from build123d import *

# Parameters (mm, degrees)
SKETCH_3_R          = 13
EXTRUDE_1_DEPTH     = 5
CUT_EXTRUDE_2_DEPTH = 2.5
SKETCH_4_R          = 10
EXTRUDE_2_DEPTH     = 15


with BuildPart() as part:
    # ｽｹｯﾁ3 → ﾎﾞｽ - 押し出し1 (new body)
    with BuildSketch(Plane.XY):
        Circle(SKETCH_3_R)
    extrude(amount=EXTRUDE_1_DEPTH)

    # ｽｹｯﾁ2 → ｶｯﾄ - 押し出し2 (cut)
    with BuildSketch(Plane.XY):
        with BuildLine():
            Line((3.75, 6.495190528), (2.463350586, 13.926501921))
            ThreePointArc((2.463350586, 13.926501921), (0, 16), (-2.463350586, 13.926501921))
            Line((-2.463350586, 13.926501921), (-3.75, 6.495190528))
            Line((-3.75, 6.495190528), (-10.829029157, 9.096575147))
            ThreePointArc((-10.829029157, 9.096575147), (-13.856406461, 8), (-13.292379743, 4.829926775))
            Line((-13.292379743, 4.829926775), (-7.5, 0))
            Line((-7.5, 0), (-13.292379743, -4.829926775))
            ThreePointArc((-13.292379743, -4.829926775), (-13.856406461, -8), (-10.829029157, -9.096575147))
            Line((-10.829029157, -9.096575147), (-3.75, -6.495190528))
            Line((-3.75, -6.495190528), (-2.463350586, -13.926501921))
            ThreePointArc((-2.463350586, -13.926501921), (0, -16), (2.463350586, -13.926501921))
            Line((2.463350586, -13.926501921), (3.75, -6.495190528))
            Line((3.75, -6.495190528), (10.829029157, -9.096575147))
            ThreePointArc((10.829029157, -9.096575147), (13.856406461, -8), (13.292379743, -4.829926775))
            Line((13.292379743, -4.829926775), (7.5, 0))
            Line((7.5, 0), (13.292379743, 4.829926775))
            ThreePointArc((13.292379743, 4.829926775), (13.856406461, 8), (10.829029157, 9.096575147))
            Line((10.829029157, 9.096575147), (3.75, 6.495190528))
        make_face()
    extrude(amount=CUT_EXTRUDE_2_DEPTH, mode=Mode.SUBTRACT)

    # ｽｹｯﾁ4 → ﾎﾞｽ - 押し出し2 (add)
    with BuildSketch(Plane.XY.offset(5)):
        Circle(SKETCH_4_R)
    extrude(amount=EXTRUDE_2_DEPTH)

    # ｽｹｯﾁ5 → 回転1 (revolve)
    with BuildSketch(Plane(origin=(0, 0, 0), x_dir=(1, 0, 0), z_dir=(0, 1, 0))):
        Polygon((0, -20), (25, -20), (25, -22), (10, -22), (10, -30), (25, -30), (25, -32), (0, -32), align=None)
    revolve(axis=Axis((0, 0, 0), (0, 0, 1)))


solid = part.part
Check sheet for the modelled part. Datum: model origin and axes. Units: mm. A direction names the side the tool comes from. Round coordinates to 2 decimals unless told otherwise and drop trailing zeros. Loops run counter-clockwise (first coordinate to the right, second up) from the corner with the lowest first, then second, coordinate; pieces in that order, holes last. Notation, with made-up numbers: M 6.5,49.5 L 24.5,49.5 A21 ccw 24.5,53.5 Z; hole C 65,72.25 d8. An arc over 180 degrees is marked long. One line per question, with ' | ' between items. Start each with the question number.
Item 1: Set-up check for faces 4 (the face through (0, -11, 30)), 5 (the face through (6.67, -7.57, 1.23)), 6 (the face through (3.218, 9.565, 1.232)): record each of +Z, -Z, +X, -X, +Y, -Y from which the full face is reachable in a straight line by a thin tool's end or side.
Item 2: Scan lines: probe 1 along Z at (x, y) = (-14, -9.5); probe 2 along Y at (x, z) = (-0.5, 29); probe 3 along X at (y, z) = (4, 3). Record each from-to range of solid material in increasing order.
Item 3: Release check for a two-part mould opening along Z. For faces 1 (the face through (0, -11, 22)), 2 (the face through (5, 10, 0)), 3 (the face through (23.846, 7.509, 31.014)) record: released by +Z, released by -Z, zero draft, split by the parting line, or undercut.
Item 4: Gauge pin test, flat ends, axial feed: pin 1 Ø5 at (y, z) = (-10, 4.5) entering from +X; pin 2 Ø4 at (y, z) = (-4.5, 16.5) entering from +X. Record the tip position at first contact, or that the pin passes through.
Item 5: Section check A-A (y = 15). Record the boundary of the cut face in (x, z).
Item 6: Section check B-B (x = -20). Record the boundary of the cut face in (y, z), and give its area (3 significant figures).
Item 7: Section check C-C (x = 0). Record the boundary of the cut face in (y, z), and give its area (3 significant figures).
Item 8: Section check D-D (y = 5). Record the boundary of the cut face in (x, z).
Worked out:
1) face 4: none | face 5: -Z, +X | face 6: -Z
2) probe 1: 20 to 22, 30 to 32 | probe 2: -9.99 to 9.99 | probe 3: -12.37 to 12.37
3) face 1: undercut | face 2: released by -Z | face 3: zero draft
4) pin 1: x = 10.62 | pin 2: x = 9.68
5) outline: M -20,20 L 20,20 L 20,22 L -20,22 Z; M -20,30 L 20,30 L 20,32 L -20,32 Z
6) outline: M -15,20 L 15,20 L 15,22 L -15,22 Z; M -15,30 L 15,30 L 15,32 L -15,32 Z | area: 120 mm^2
7) outline: M -25,20 L -10,20 L -10,5 L -13,5 L -13,2.5 L 13,2.5 L 13,5 L 10,5 L 10,20 L 25,20 L 25,22 L 10,22 L 10,30 L 25,30 L 25,32 L -25,32 L -25,30 L -10,30 L -10,22 L -25,22 Z | area: 725 mm^2
8) outline: M -24.49,20 L -8.66,20 L -8.66,5 L -12,5 L -12,2.5 L 12,2.5 L 12,5 L 8.66,5 L 8.66,20 L 24.49,20 L 24.49,22 L 8.66,22 L 8.66,30 L 24.49,30 L 24.49,32 L -24.49,32 L -24.49,30 L -8.66,30 L -8.66,22 L -24.49,22 Z
